Source: CAD feature listing. Evaluate the final solid. Frame: model axes, mm. A direction names the side the tool comes from. Coordinates: 2 decimals unless noted, no trailing zeros. Order: outer loops, then holes, each group sorted by start corner. A loop starts at its lowest first (then second) coordinate and runs counter-clockwise, first axis right, second up.
```python
from build123d import *

# Parameters (mm, degrees)
F0_R     = 25.4
F1_DEPTH = 12.7
F2_DEPTH = 25.4
F3_R     = 22.051706
F4_DEPTH = 50.8


with BuildPart() as f1:
    # F0 (on Top) → F1 (new body)
    with BuildSketch(Plane.XY):
        with BuildLine():
            Line((3.983806, 43.125236), (-129.739803, 43.125236))
            Line((-129.739803, 43.125236), (-129.739803, -7.674764))
            Line((-129.739803, -7.674764), (-129.739803, -58.474764))
            Line((-129.739803, -58.474764), (-15.439803, -58.474764))
            Line((-15.439803, -58.474764), (73.460197, -58.474764))
            ThreePointArc((73.460197, -58.474764), (46.476896, -2.371791), (3.983806, 43.125236))
        make_face()
        with Locations((-15.439803, -7.674764)):
            Circle(F0_R, mode=Mode.SUBTRACT)
        with BuildLine():
            ThreePointArc((-21.157369, 60.119772), (-8.273827, 52.085478), (3.983806, 43.125236))
            Line((3.983806, 43.125236), (73.460197, 43.125236))
            ThreePointArc((73.460197, 43.125236), (33.692598, 82.321217), (-21.157369, 92.774352))
            Line((-21.157369, 92.774352), (-21.157369, 60.119772))
        make_face()
        with BuildLine():
            Line((73.460197, 43.125236), (3.983806, 43.125236))
            ThreePointArc((3.983806, 43.125236), (46.476896, -2.371791), (73.460197, -58.474764))
            Line((73.460197, -58.474764), (73.460197, 43.125236))
        make_face()
        Polygon((-49.437065, 43.792482), (-21.157369, 60.119772), (-21.157369, 92.774352), (-49.437065, 109.101642), (-77.71676, 92.774352), (-77.71676, 60.119772), align=None)
    extrude(amount=F1_DEPTH)

    # F0 (on Top) → F2 (join)
    with BuildSketch(Plane.XY):
        with BuildLine():
            Line((3.983806, 43.125236), (-129.739803, 43.125236))
            Line((-129.739803, 43.125236), (-129.739803, -7.674764))
            Line((-129.739803, -7.674764), (-129.739803, -58.474764))
            Line((-129.739803, -58.474764), (-15.439803, -58.474764))
            Line((-15.439803, -58.474764), (73.460197, -58.474764))
            ThreePointArc((73.460197, -58.474764), (46.476896, -2.371791), (3.983806, 43.125236))
        make_face()
        with Locations((-15.439803, -7.674764)):
            Circle(F0_R, mode=Mode.SUBTRACT)
        with BuildLine():
            ThreePointArc((-21.157369, 60.119772), (-8.273827, 52.085478), (3.983806, 43.125236))
            Line((3.983806, 43.125236), (73.460197, 43.125236))
            ThreePointArc((73.460197, 43.125236), (33.692598, 82.321217), (-21.157369, 92.774352))
            Line((-21.157369, 92.774352), (-21.157369, 60.119772))
        make_face()
        with BuildLine():
            Line((73.460197, 43.125236), (3.983806, 43.125236))
            ThreePointArc((3.983806, 43.125236), (46.476896, -2.371791), (73.460197, -58.474764))
            Line((73.460197, -58.474764), (73.460197, 43.125236))
        make_face()
        Polygon((-49.437065, 43.792482), (-21.157369, 60.119772), (-21.157369, 92.774352), (-49.437065, 109.101642), (-77.71676, 92.774352), (-77.71676, 60.119772), align=None)
    extrude(amount=F2_DEPTH)

    # F3 (on Front) → F4 (join)
    with BuildSketch(Plane.XZ):
        with Locations((-100.670184, 47.124073)):
            Circle(F3_R)
    extrude(amount=F4_DEPTH)


solid = f1.part
```
1. Pin query (flat end, axial travel): P1, Ø20.5, axis at y = 70.5, z = 8, coming from the -X side; P2, Ø22, axis at x = -106, z = 40.5, coming from the +Y side; P3, Ø13, axis at x = -110.5, z = 45.5, coming from the -Y side. Return the tip coordinate at first contact, or that it passes through.
Findings:
P1: stops at x = -77.72
P2: stops at y = 0
P3: stops at y = -50.8
2. Section query D-D on z = 20.5. Return loops of the section in (x, y).
Findings:
outline: (-129.74, -58.47) - (73.46, -58.47) - (73.46, 43.13) arc R96.05 ccw to (-21.16, 92.77) - (-49.44, 109.1) - (-77.72, 92.77) - (-77.72, 60.12) - (-49.44, 43.79) - (-21.16, 60.12) arc R206.27 cw to (3.98, 43.13) - (-129.74, 43.13) - close; hole circle Ø50.8 at (-15.44, -7.67)
3. Access query for faces 4 (the face through (-35.5, 51.84, 12.52)), 5 (the face through (-101, -50.8, 48)), 6 (the face through (-77.717, 77, 13)). Directions: +Z, -Z, +X, -X, +Y, -Y. A direction counts if a zero-diameter tool reaches every point of the face in a straight line with its end or side. Return the directions, or none.
Findings:
face 4: +Z, -Z
face 5: +Z, +X, -X, -Y
face 6: +Z, -Z, -X, +Y
4. Draft query along Z for faces 1 (the face through (-99.754, -25.044, 69.157)), 2 (the face through (-30, 26, 0)), 3 (the face through (-101, 0, 48)). Return one class per face: released by +Z, released by -Z, zero draft, split by the parting line, or undercut.
Findings:
face 1: undercut
face 2: released by -Z
face 3: zero draft
5. Section query B-B on y = 53.5. Return loops of the section in (x, z).
Findings:
outline: (-66.25, 0) - (-32.62, 0) - (-32.62, 25.4) - (-66.25, 25.4) - close; (-10.39, 0) - (66.93, 0) - (66.93, 25.4) - (-10.39, 25.4) - close
6. Section query A-A on x = -71.5. Return loops of the section in (y, z).
Findings:
outline: (-58.47, 0) - (43.13, 0) - (43.13, 25.4) - (-58.47, 25.4) - close; (56.53, 0) - (96.36, 0) - (96.36, 25.4) - (56.53, 25.4) - close
7. Ray query, line 1 (Y direction, x = -24, z = 18); line 2 (Z direction, x = -37.5, y = 80.5); line 3 (Y direction, x = -85, z = 39). Return the intervals inside material, ascending.
Findings:
line 1: y = -58.47 to -31.59, 16.24 to 43.13, 58.48 to 94.42
line 2: z = 0 to 25.4
line 3: y = -50.8 to 0
8. Section query C-C on x = -5.5. Return loops of the section in (y, z).
Findings:
outline: (-58.47, 0) - (-31.05, 0) - (-31.05, 25.4) - (-58.47, 25.4) - close; (15.7, 0) - (43.13, 0) - (43.13, 25.4) - (15.7, 25.4) - close; (50.18, 0) - (93.17, 0) - (93.17, 25.4) - (50.18, 25.4) - close
